from build123d import *

# Parameters (mm, degrees)
SKETCH1_R                                       = 5
EXTRUDE1_DEPTH                                  = 4
CSK_FOR_M2_OVAL_HEAD_MACHINE_SCREW1_D           = 2.4
CSK_FOR_M2_OVAL_HEAD_MACHINE_SCREW1_CSINK_D     = 4.4
CSK_FOR_M2_OVAL_HEAD_MACHINE_SCREW1_CSINK_ANGLE = 90
CIRPATTERN2_COUNT                               = 3
EXTRUDE4_START                                  = 4.45086
EXTRUDE4_DEPTH                                  = 7.205259
EXTRUDE5_START                                  = 4.330127
EXTRUDE5_DEPTH                                  = 7.205258
EXTRUDE6_START                                  = 4.330127
EXTRUDE6_DEPTH                                  = 7.205258


with BuildPart() as part:
    # Sketch1 → Extrude1 (new body)
    with BuildSketch(Plane(origin=(0, 0, 0), x_dir=(1, 0, 0), z_dir=(0, 1, 0))):
        with BuildLine():
            Line((-3.89089061, 3.146959138), (-2.360502052, 0.4962484))
            ThreePointArc((-2.360502052, 0.4962484), (-2.104118872, -0.718531203), (-2.613989574, -1.850544314))
            ThreePointArc((-2.613989574, -1.850544314), (-2.994220859, -5.370733384), (0.244467944, -6.801537968))
            ThreePointArc((0.244467944, -6.801537968), (1.479755407, -6.925983542), (2.403593813, -7.75540769))
            Line((2.403593813, -7.75540769), (3.933982371, -10.406118428))
            ThreePointArc((3.933982371, -10.406118428), (6.099045881, -11.656118428), (8.26410939, -10.406118428))
            Line((8.26410939, -10.406118428), (9.794497948, -7.75540769))
            ThreePointArc((9.794497948, -7.75540769), (10.718336354, -6.925983542), (11.953623817, -6.801537968))
            ThreePointArc((11.953623817, -6.801537968), (15.192312621, -5.370733384), (14.812081336, -1.850544314))
            ThreePointArc((14.812081336, -1.850544314), (14.302210633, -0.718531203), (14.558593813, 0.4962484))
            Line((14.558593813, 0.4962484), (16.088982371, 3.146959138))
            ThreePointArc((16.088982371, 3.146959138), (16.088982371, 5.646959138), (13.923918862, 6.896959138))
            Line((13.923918862, 6.896959138), (10.863141746, 6.896959138))
            ThreePointArc((10.863141746, 6.896959138), (9.68292016, 7.282314592), (8.9575034, 8.289882129))
            ThreePointArc((8.9575034, 8.289882129), (6.099045881, 10.379266616), (3.240588362, 8.289882129))
            ThreePointArc((3.240588362, 8.289882129), (2.515171602, 7.282314592), (1.334950016, 6.896959138))
            Line((1.334950016, 6.896959138), (-1.7258271, 6.896959138))
            ThreePointArc((-1.7258271, 6.896959138), (-3.89089061, 5.646959138), (-3.89089061, 3.146959138))
        make_face()
        with Locations((6.099045881, -0.120733384)):
            Circle(SKETCH1_R, mode=Mode.SUBTRACT)
    extrude(amount=EXTRUDE1_DEPTH)

    # CSK for M2 Oval Head Machine Screw1 (through all)
    with Locations(Plane(origin=(-0.396144648, 0, 3.870733384), x_dir=(0, 0, -1), z_dir=(0, -1, 0))):
        with Locations((0, 0)):
            csk_for_m2_oval_head_machine_screw1 = CounterSinkHole(CSK_FOR_M2_OVAL_HEAD_MACHINE_SCREW1_D / 2, CSK_FOR_M2_OVAL_HEAD_MACHINE_SCREW1_CSINK_D / 2, counter_sink_angle=CSK_FOR_M2_OVAL_HEAD_MACHINE_SCREW1_CSINK_ANGLE)

    # CirPattern2: CSK for M2 Oval Head Machine Screw1 ×3 about axis
    cirpattern2_axis = Axis((6.099045881, 0, 0.120733384), (0, 1, 0))
    for i in range(1, CIRPATTERN2_COUNT):
        add(csk_for_m2_oval_head_machine_screw1.rotate(cirpattern2_axis, i * 360 / CIRPATTERN2_COUNT), mode=Mode.SUBTRACT)

    # GrooveSketch → Extrude4 (cut)
    with BuildSketch(Plane.XY.offset(EXTRUDE4_START)):
        Polygon((34.668922444, -26.069876563), (8.599045881, 0), (6.099045881, 2.5), (3.599045881, 0), (-22.470830682, -26.069876563), (-22.470830682, -99.806622573), (34.668922444, -99.806622573), align=None)
    extrude(amount=EXTRUDE4_DEPTH, mode=Mode.SUBTRACT)

    # Sketch9 → Extrude5 (cut)
    with BuildSketch(Plane(origin=(4.6265635, 0, 2.671147682), x_dir=(-0.5, 0, 0.866025404), z_dir=(-0.866025404, 0, -0.5)).offset(EXTRUDE5_START)):
        Polygon((32.223222882, -32.668187644), (-0.444964763, 0), (-2.944964763, 2.5), (-5.444964763, 0), (-38.113152407, -32.668187644), (-38.113152407, -125.067775694), (32.223222882, -125.067775694), align=None)
    extrude(amount=EXTRUDE5_DEPTH, mode=Mode.SUBTRACT)

    # Sketch10 → Extrude6 (cut)
    with BuildSketch(Plane(origin=(4.522005322, 0, -2.61078099), x_dir=(-0.5, 0, -0.866025404), z_dir=(0.866025404, 0, -0.5)).offset(EXTRUDE6_START)):
        Polygon((32.014106526, -32.668187644), (-0.654081118, 0), (-3.154081118, 2.5), (-5.654081118, 0), (-38.322268763, -32.668187644), (-38.322268763, -125.067775694), (32.014106526, -125.067775694), align=None)
    extrude(amount=EXTRUDE6_DEPTH, mode=Mode.SUBTRACT)


solid = part.part
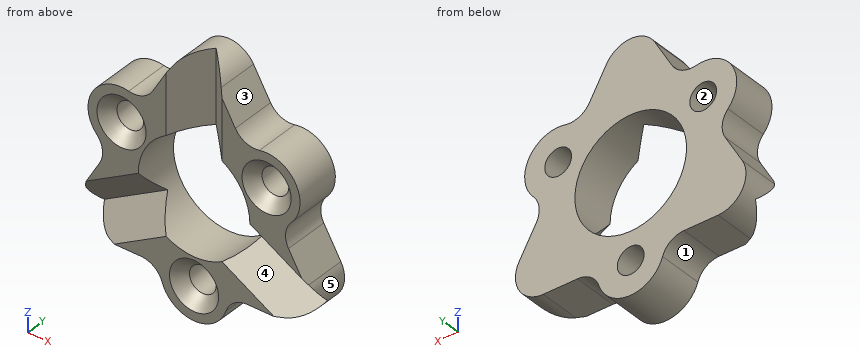
Read the model definition and answer for the solid it produces. Units are mm, in the model's axes. Face numbers are marked on the shaded views. A direction names the side the tool comes from. Give positions to 0.01 mm unless a question says otherwise; leave off trailing zeros. Write each loop counter-clockwise with the first axis right and the second up, starting at its lowest first coordinate (ties: lowest second). Pieces come first, ordered by that corner, then holes. Notation, with made-up numbers: (79.5, 6) - (127.5, 6) arc R34 cw to (127.5, 40) - close; hole circle Ø7 at (24.25, 32.25). An arc over 180 degrees is marked (long way). Use CSV: the item, a comma, the result in double quotes. Start each with the question number.
Item 1: The mould has two halves that part along X. Classify the marked faces 1, 2 and 3: pulls with the +X half, pulls with the -X half, needs draft (parallel to the pull), parting line crosses it, or undercut.
Item 2: The part is cut by section A-A, the plane x = 9.25. Give the vertices of the cut face in (y, z).
Item 3: Flat-ended cylindrical pins translate along their axes: P1, Ø0.9, axis at x = 0.5, y = 2, coming from the -Z side; P2, Ø1, axis at x = 10, z = -4.5, coming from the -Y side; P3, Ø3, axis at x = -0.4, z = 3.87, coming from the -Y side. Find the tip coordinate at first contact, or state that the pin passes through.
Item 4: The part is cut by section D-D, the plane z = 6.5. Give the vertices of the cut face in (x, y).
Item 5: Consider line 1 (Z direction, x = 11.75, y = 0.45); line 2 (Z direction, x = 6, y = 1.3); line 3 (Z direction, x = 14.75, y = 1.05). Determine where each line is inside the solid, lowest interval first.
Item 6: For the marked faces 4 and 5, determine the directions among +Z, -Z, +X, -X, +Y, -Y from which every point of the face is accessible in a straight line to the end or side of a thin tool.
Item 7: The part is cut by section C-C, the plane z = -4.5. Give the vertices of the cut face in (x, y).
Item 8: The part is cut by section B-B, the plane y = 3.65. Give the vertices of the cut face in (x, z), and give its area (3 significant figures).
Taken from the geometry:
1,face 1,"pulls with the -X half"
1,face 2,"undercut"
1,face 3,"pulls with the +X half"
2,outline,"(0, -7.71) - (4, -7.71) - (4, -3.76) - (0.71, -3.76) - (0, -4.59) - close; (0, 4) - (4, 4) - (4, 8.7) - (0, 8.7) - close"
3,P1,"z = -6.9"
3,P2,"y = 0"
3,P3,"y = 0.7"
4,outline,"(-1.84, 0) - (3.6, 0) - (6.1, 2.5) - (8.6, 0) - (14.04, 0) - (14.04, 4) - (-1.84, 4) - close"
5,line 1,"-6.9 to -5.51, -0.77 to 2.34, 5.4 to 6.77"
5,line 2,"-10.38 to -8.58, -6.18 to -4.88"
5,line 3,"-6.76 to -6.55, -3.2 to -0.83, 1.78 to 5.96"
6,face 4,"-Y"
6,face 5,"+X, +Y, -Y"
7,outline,"(-4.22, 1.34) - (-1.9, 2.5) - (3.1, 0) - (4.19, 0) - (4.19, 4) - (-4.22, 4) - close; (8.01, 0) - (9.1, 0) - (14.1, 2.5) - (16.42, 1.34) - (16.42, 4) - (8.01, 4) - close"
8,outline,"(-3.89, -3.15) arc R2.5 ccw to (-1.73, -6.9) - (1.33, -6.9) arc R2 cw to (3.24, -8.29) arc R3 ccw to (8.96, -8.29) arc R2 cw to (10.86, -6.9) - (13.92, -6.9) arc R2.5 ccw to (16.09, -3.15) - (14.56, -0.5) arc R2 cw to (14.81, 1.85) arc R3 ccw to (11.95, 6.8) arc R2 cw to (9.79, 7.76) - (8.26, 10.41) arc R2.5 ccw to (3.93, 10.41) - (2.4, 7.76) arc R2 cw to (0.24, 6.8) arc R3 ccw to (-2.61, 1.85) arc R2 cw to (-2.36, -0.5) - close; hole circle Ø2.4 at (-0.4, 3.87); hole circle Ø10 at (6.1, 0.12); hole circle Ø2.4 at (6.1, -7.38); hole circle Ø2.4 at (12.59, 3.87)"
8,area,"205 mm2"
